Autodesk Fusion 360 part; units mm, degrees
sketch "Sketch1" plane through (0, 0, 0) normal (0, 0, 1) x (1, 0, 0)
  line L0 (12.5, -12.5) -> (-12.5, -12.5)
  line L1 (-12.5, -12.5) -> (-12.5, 12.5)
  line L2 (-12.5, 12.5) -> (12.5, 12.5)
  line L3 (12.5, 12.5) -> (12.5, -12.5)
  line L4 (12.5, -12.5) -> (-12.5, 12.5) construction
  line L5 (-12.5, -12.5) -> (12.5, 12.5) construction
  line L6 (10.05, -10.05) -> (-10.05, -10.05)
  line L7 (-10.05, -10.05) -> (-10.05, 10.05)
  line L8 (-10.05, 10.05) -> (10.05, 10.05)
  line L9 (10.05, 10.05) -> (10.05, -10.05)
  line L10 (10.05, -10.05) -> (-10.05, 10.05) construction
  line L11 (-10.05, -10.05) -> (10.05, 10.05) construction
  dimension "d3" = 25
  dimension "d4" = 25
  dimension "d5" = 20.1
  dimension "d6" = 20.1
extrude "Extrude1" add sketch "Sketch1" along normal blind 15 makes body 1
sketch "Sketch2" plane through (0, 0, 15) normal (0, 0, 1) x (-1, 0, 0)
  line L0 (10.05, -10.05) -> (-10.05, -10.05)
  line L1 (-10.05, -10.05) -> (-10.05, 10.05)
  line L2 (-10.05, 10.05) -> (10.05, 10.05)
  line L3 (10.05, 10.05) -> (10.05, -10.05)
  line L4 (-12.5, -12.5) -> (12.5, -12.5)
  line L5 (12.5, -12.5) -> (12.5, 12.5)
  line L6 (12.5, 12.5) -> (-12.5, 12.5)
  line L7 (-12.5, 12.5) -> (-12.5, -12.5)
  line L8 (12.5, -12.5) -> (7.5, -12.5)
  line L9 (7.5, -12.5) -> (7.5, 12.5)
  line L10 (7.5, 12.5) -> (12.5, 12.5)
  line L11 (12.5, 12.5) -> (12.5, -12.5)
  line L12 (-12.5, -12.5) -> (-7.5, -12.5)
  line L13 (-7.5, -12.5) -> (-7.5, 12.5)
  line L14 (-7.5, 12.5) -> (-12.5, 12.5)
  line L15 (-12.5, 12.5) -> (-12.5, -12.5)
  dimension "d9" = 5
  dimension "d10" = 5
extrude "Extrude2" add sketch "Sketch2" along normal blind 25 contours L0 L2 L3 L4 L5 L6 L8 L9 L10 L11 | L0 L2 L3 L9 | L0 L1 L2 L4 L6 L7 L12 L13 L14 L15 | L0 L1 L2 L13 bodies 1
sketch "Sketch3" plane through (-12.5, 0, 0) normal (-1, 0, 0) x (0, -1, 0)
  line L0 (-12.5, 0) -> (12.5, 0)
  line L1 (12.5, 0) -> (12.5, 40)
  line L2 (12.5, 40) -> (-12.5, 40)
  line L3 (-12.5, 40) -> (-12.5, 0)
  line L4 (0, 40) -> (0, 0) construction
  line L5 (4, 32.3094) -> (0, 34.6188)
  line L6 (0, 34.6188) -> (-4, 32.3094)
  line L7 (-4, 32.3094) -> (-4, 27.6906)
  line L8 (-4, 27.6906) -> (0, 25.3812)
  line L9 (0, 25.3812) -> (4, 27.6906)
  line L10 (4, 27.6906) -> (4, 32.3094)
  point P0 (0, 30)
  point P1 (0, 30)
  dimension "d13" = 10
  dimension "d27" = 4
hole "Hole1" at (-12.5, 0, 30) direction (1, 0, 0) diameter 5.5 end through all bodies 1 1
sketch "Sketch4" plane through (-7.5, 0, 0) normal (1, 0, 0) x (0, 1, 0)
  circle A0 centre (0, 30) radius 2.75
  line L0 (10.05, 15) -> (12.5, 15)
  line L1 (12.5, 15) -> (12.5, 40)
  line L2 (12.5, 40) -> (-12.5, 40)
  line L3 (-12.5, 40) -> (-12.5, 15)
  line L4 (-12.5, 15) -> (-10.05, 15)
  line L5 (-10.05, 15) -> (10.05, 15)
  circle A1 centre (0, 30) radius 4
  dimension "d17" = 8
sketch "Sketch5" plane through (7.5, 0, 0) normal (-1, 0, 0) x (0, -1, 0)
  circle A0 centre (0, 30) radius 2.75
  line L0 (-12.5, 15) -> (-10.05, 15)
  line L1 (-10.05, 15) -> (10.05, 15)
  line L2 (10.05, 15) -> (12.5, 15)
  line L3 (12.5, 15) -> (12.5, 40)
  line L4 (12.5, 40) -> (-12.5, 40)
  line L5 (-12.5, 40) -> (-12.5, 15)
  circle A1 centre (0, 30) radius 4
  dimension "d22" = 8
extrude "Extrude3" add sketch "Sketch4" along normal blind 3.275 contours A1 bodies 1
extrude "Extrude4" add sketch "Sketch5" along normal blind 3.275 contours A1 bodies 1
fillet "Fillet2" radius 3 2 edges at (7.5, 3.7293, 31.4465) (-7.5, -3.7293, 31.4465) on bodies 1
extrude "Extrude5" cut sketch "Sketch3" against normal blind 3.5 contours L5 L6 L7 L8 L9 L10 bodies 1
sketch "Sketch6" plane through (0, 0, 0) normal (0, 0, -1) x (1, 0, 0)
  line L0 (10.05, -10.05) -> (-10.05, -10.05)
  line L1 (-10.05, -10.05) -> (-10.05, 10.05)
  line L2 (-10.05, 10.05) -> (10.05, 10.05)
  line L3 (10.05, 10.05) -> (10.05, -10.05)
  line L4 (-12.5, -12.5) -> (12.5, -12.5)
  line L5 (12.5, -12.5) -> (12.5, 12.5)
  line L6 (12.5, 12.5) -> (-12.5, 12.5)
  line L7 (-12.5, 12.5) -> (-12.5, -12.5)
  line L8 (-7.5, -10.05) -> (-7.5, 10.05)
  line L9 (7.5, -10.05) -> (7.5, 10.05)
  line L10 (-12.5, 12.5) -> (-6, 19)
  line L11 (-6, 19) -> (0, 19)
  line L12 (0, 19) -> (0, 17)
  line L13 (-10.05, 10.05) -> (-3.1, 17)
  line L14 (0, 17) -> (-3.1, 17)
  line L15 (-7.6, 10.05) -> (-7.6, 12.5)
  line L16 (0, -1.75) -> (0, -22.5)
  line L17 (0, 17) -> (3.1, 17)
  line L18 (6, 19) -> (0, 19)
  line L19 (0, 19) -> (0, 17)
  line L20 (10.05, 10.05) -> (3.1, 17)
  line L21 (12.5, 12.5) -> (6, 19)
  line L22 (7.6, 10.05) -> (7.6, 12.5)
  line L23 (1.75, 0) -> (22.5, 0)
  line L24 (10.05, -10.05) -> (3.1, -17)
  line L25 (7.6, -10.05) -> (7.6, -12.5)
  line L26 (12.5, -12.5) -> (6, -19)
  line L27 (6, -19) -> (0, -19)
  line L28 (0, -17) -> (3.1, -17)
  line L29 (0, -17) -> (-3.1, -17)
  line L30 (-6, -19) -> (0, -19)
  line L31 (-12.5, -12.5) -> (-6, -19)
  line L32 (-10.05, -10.05) -> (-3.1, -17)
  line L33 (-7.6, -10.05) -> (-7.6, -12.5)
  dimension "d30" = 2
  dimension "d31" = 45
  dimension "d37" = 6.5
extrude "Extrude6" cut sketch "Sketch6" against normal blind 15 contours L0 L4 L16 L25 | L0 L4 L16 L33 | L2 L6 L15 L22 bodies 1 makes body 2 at (-12.5, 0, 8.4604)
extrude "Extrude7" add sketch "Sketch6" against normal blind 15 contours L4 L16 L24 L26 L27 L28 | L6 L12 L17 L18 L19 L20 L21 | L4 L16 L29 L30 L31 L32 | L6 L10 L11 L12 L13 L14 L19 bodies 1 2
chamfer "Chamfer1" distance 8 angle 45 4 edges at (10, -12.5, 40) (-10, -12.5, 40) (-10, 12.5, 40) (10, 12.5, 40) on bodies 1 2
fillet "Fillet1" [suppressed]
The model under review builds one solid part; all positions refer to its coordinate system, in mm. A direction names the side the tool comes from. Give positions to 0.01 mm unless a question says otherwise; leave off trailing zeros. Write each loop counter-clockwise with the first axis right and the second up, starting at its lowest first coordinate (ties: lowest second). Pieces come first, ordered by that corner, then holes.
(1) Tool access review of faces 4 (the flat face through (-11, -4, 30)), 5 (the flat face through (9, -10.05, 7)), 6 (the flat face through (5.4, -14.7, 7.4)): name each direction out of +Z, -Z, +X, -X, +Y, -Y from which nothing blocks a thin tool from reaching the whole face with its end or side.
(2) The part is to be moulded in two halves that separate along Y. For faces 1 (the flat face through (-7.6, -11, 7)), 2 (the flat face through (-10, 8.4, 36.1)), 3 (the flat face through (10, -8.4, 36.1)), say which applies: released by +Y, released by -Y, zero draft, split by the parting line, or undercut.
(3) For P1, Ø9, axis at y = 1.5, z = 28, coming from the -X side; P2, Ø2.5, axis at x = -9.5, z = 5.5, coming from the -Y side; P3, Ø1, axis at x = -7.5, z = 20, coming from the +Y side; P4, Ø2, axis at x = -5, y = 14.5, coming from the +Z side, all flat-tipped, find the tip position at first contact; note any pin that passes through.
(4) Consider section B-B, the plane z = 30. Give the number of separate pieces and of enclosed holes in the cut face, and give its area (3 significant figures).
(5) Consider section A-A, the plane y = -13. Give the boundary of the cut face in (x, z).
(6) Consider section D-D, the plane z = 17.5. Give the boundary of the cut face in (x, y).
(7) To check wall thickness, follow L1, parallel to Z at x = -7.95, y = 0; L2, parallel to Z at x = -8, y = -1.5; L3, parallel to Y at x = 10, z = 30. State the ranges of each line that lie inside material, in increasing order.
(8) Consider section C-C, the plane x = -6.5. Give the boundary of the cut face in (y, z).
Returned:
1. face 4: -X
1. face 5: -Z
1. face 6: +Z, -Z
2. face 1: undercut
2. face 2: released by +Y
2. face 3: released by -Y
3. P1: stops at x = -12.5
3. P2: stops at y = -16.75
3. P3: stops at y = 12.5
3. P4: stops at z = 15
4. separate pieces: 4
4. enclosed holes: 0
4. area: 210 mm2
5. outline: (-12, 0) - (-7.1, 0) - (-7.1, 15) - (-12, 15) - close; (7.1, 0) - (12, 0) - (12, 15) - (7.1, 15) - close
6. outline: (-12.5, -12.5) - (-7.5, -12.5) - (-7.5, 12.5) - (-12.5, 12.5) - close; (7.5, -12.5) - (12.5, -12.5) - (12.5, 12.5) - (7.5, 12.5) - close
7. L1: z = 15 to 27.25, 32.75 to 40
7. L2: z = 15 to 27.7, 32.3 to 40
7. L3: y = -12.5 to -2.75, 2.75 to 12.5
8. outline: (-18.5, 0) - (-13.6, 0) - (-13.6, 15) - (-18.5, 15) - close; circle Ø9.53 at (0, 30); (13.6, 0) - (18.5, 0) - (18.5, 15) - (13.6, 15) - close; hole circle Ø5.5 at (0, 30)
